Here's the drawing with two shaded views (mm, measured from the low corner). I have some questions. A direction names the side the tool comes from. Round coordinates to 2 decimals unless told otherwise and drop trailing zeros. Order: outer loops, then holes, each group sorted by start corner. A loop starts at its lowest first (then second) coordinate and runs counter-clockwise, first axis right, second up. Notation, with made-up numbers: (-12, 38.5) -> (3, 38.5) arc R28 cw to (3, 75.5) -> close; hole circle Ø8 at (88.25, -2.5). An arc over 180 degrees is marked (long way). Answer in a Markdown table with one row per item.
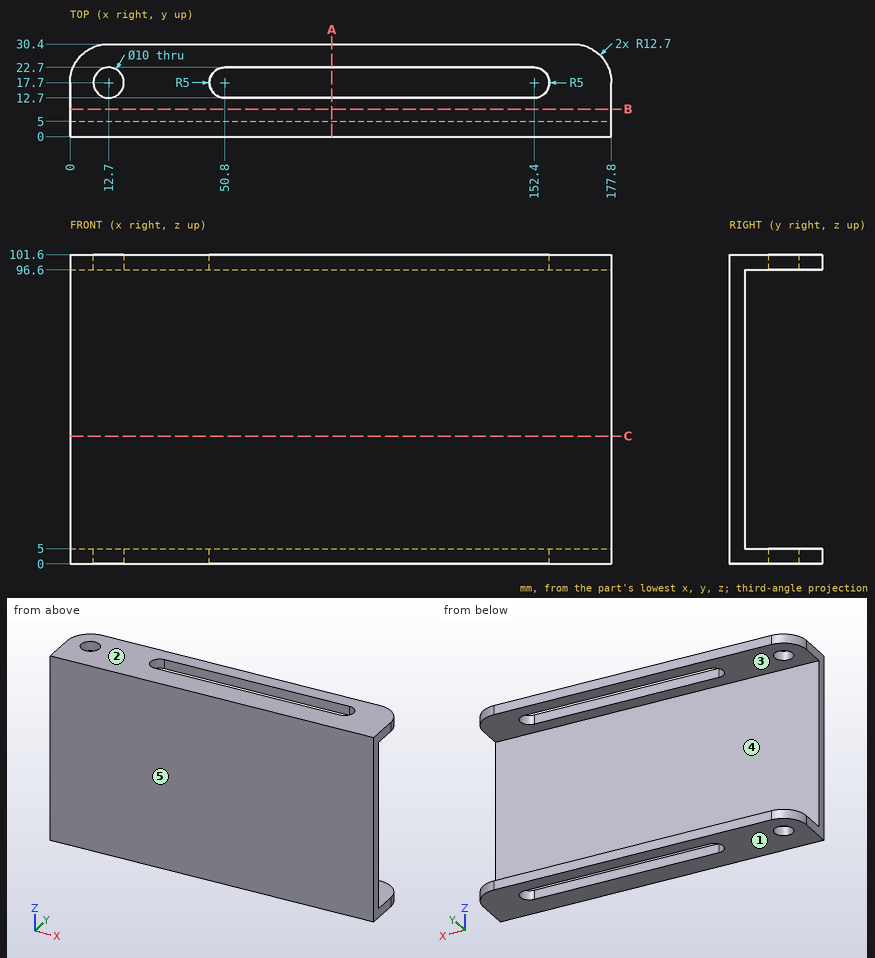
1. Suppose I cut it at B-B on y = 9. Write out the boundary of the cut face in (x, z), then the cut area to 3 significant figures.
Numbers:
| item | result |
|---|---|
| outline | (0, 0) -> (177.8, 0) -> (177.8, 5) -> (0, 5) -> close; (0, 96.6) -> (177.8, 96.6) -> (177.8, 101.6) -> (0, 101.6) -> close |
| area | 1,780 mm2 |
2. For the marked faces 4 and 5, which set-ups out of +Z, -Z, +X, -X, +Y, -Y let a thin tool reach every point of the face, with its end or its side?
Numbers:
| item | result |
|---|---|
| face 4 | +X, -X, +Y |
| face 5 | +Z, -Z, +X, -X, -Y |
3. Suppose I cut it at C-C on z = 42. Write out the boundary of the cut face in (x, y), then the cut area to 3 significant figures.
Numbers:
| item | result |
|---|---|
| outline | (0, 0) -> (177.8, 0) -> (177.8, 5) -> (0, 5) -> close |
| area | 889 mm2 |
4. Please list where these lines run through material, in increasing order: line 1 along Z through (x, y) = (138, 7); line 2 along X through (y, z) = (17, 99); line 3 along Y through (x, z) = (60.5, 63.5).
Numbers:
| item | result |
|---|---|
| line 1 | z = 0 to 5, 96.6 to 101.6 |
| line 2 | x = 0 to 7.75, 17.65 to 45.85, 157.35 to 177.8 |
| line 3 | y = 0 to 5 |
5. For pin 1 Ø10 at (x, z) = (19.5, 76) entering from -Y; pin 2 Ø6 at (x, y) = (145, 17) entering from -Z, each with a flat end and sliding along its axis, tell me the tip position at first contact or that it passes through.
Numbers:
| item | result |
|---|---|
| pin 1 | stops at y = 0 |
| pin 2 | passes through |
6. We'd pull the mould along Z, two halves only. Please class the marked faces 1, 2 and 3: released by +Z, released by -Z, zero draft, split by the parting line, or undercut.
Numbers:
| item | result |
|---|---|
| face 1 | released by -Z |
| face 2 | released by +Z |
| face 3 | undercut |
7. Suppose I cut it at A-A on x = 86. Write out the boundary of the cut face in (y, z), then the cut area to 3 significant figures.
Numbers:
| item | result |
|---|---|
| outline | (0, 0) -> (12.7, 0) -> (12.7, 5) -> (5, 5) -> (5, 96.6) -> (12.7, 96.6) -> (12.7, 101.6) -> (0, 101.6) -> close; (22.7, 0) -> (30.4, 0) -> (30.4, 5) -> (22.7, 5) -> close; (22.7, 96.6) -> (30.4, 96.6) -> (30.4, 101.6) -> (22.7, 101.6) -> close |
| area | 662 mm2 |
